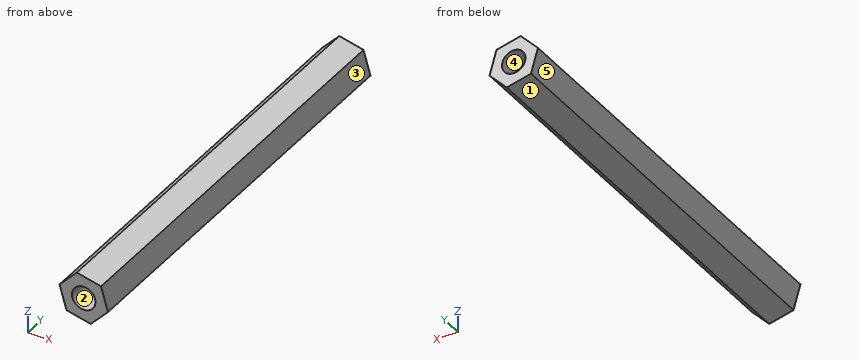
from build123d import *

# Parameters (mm, degrees)
BOSS_EXTRUDE1_DEPTH = 63.5
SKETCH2_R           = 1.7272
CUT_EXTRUDE1_DEPTH  = 9.525
SKETCH3_R           = 1.7272
CUT_EXTRUDE2_DEPTH  = 9.525


with BuildPart() as part:
    # Sketch1 → Boss-Extrude1 (new body)
    with BuildSketch(Plane(origin=(0, 0, 0), x_dir=(1, 0, 0), z_dir=(0, 1, 0))):
        Polygon((-2.767735883, 3.334911674), (-1.744793251, 6.855482892), (-4.282226046, 9.501662807), (-7.842601473, 8.627271504), (-8.865544105, 5.106700285), (-6.32811131, 2.46052037), align=None)
    extrude(amount=BOSS_EXTRUDE1_DEPTH)

    # Sketch2 → Cut-Extrude1 (cut)
    with BuildSketch(Plane(origin=(0, 63.5, 0), x_dir=(1, 0, 0), z_dir=(0, 1, 0))):
        with Locations((-5.305168678, 5.981091589)):
            Circle(SKETCH2_R)
    extrude(amount=-CUT_EXTRUDE1_DEPTH, mode=Mode.SUBTRACT)

    # Sketch3 → Cut-Extrude2 (cut)
    with BuildSketch(Plane.XZ):
        with Locations((-5.305168678, -5.981091589)):
            Circle(SKETCH3_R)
    extrude(amount=-CUT_EXTRUDE2_DEPTH, mode=Mode.SUBTRACT)


solid = part.part
Design review of the part built by this model. Coordinates are the model's own, in mm. Face numbers are marked on the shaded views. A direction names the side the tool comes from. Coordinates: 2 decimals unless noted, no trailing zeros. Order: outer loops, then holes, each group sorted by start corner. A loop starts at its lowest first (then second) coordinate and runs counter-clockwise, first axis right, second up. Notation, with made-up numbers: (2.25, 33) -> (42.25, 33) arc R16 ccw to (42.25, 41) -> close; hole circle Ø4 at (80, -0.5). An arc over 180 degrees is marked (long way). One line per item, written item: value.
1) We need section B-B, the plane x = -5. Give the boundary of the cut face in (y, z) (3 decimals).
Output values:
outline: (0, -9.325) -> (63.5, -9.325) -> (63.5, -7.681) -> (53.975, -7.681) -> (53.975, -4.281) -> (63.5, -4.281) -> (63.5, -2.787) -> (0, -2.787) -> (0, -4.281) -> (9.525, -4.281) -> (9.525, -7.681) -> (0, -7.681) -> close
2) We need section A-A, the plane y = 49.5. Give the boundary of the cut face in (x, z), then the cut area to 3 significant figures.
Output values:
outline: (-8.87, -5.11) -> (-7.84, -8.63) -> (-4.28, -9.5) -> (-1.74, -6.86) -> (-2.77, -3.33) -> (-6.33, -2.46) -> close
area: 34.9 mm2
3) To check wall thickness, follow probe 1 along Y at (x, z) = (-5, -7) (3 decimals); probe 2 along X at (y, z) = (55.5, -7.25); probe 3 along Z at (x, y) = (-6.25, 60.5). State the ranges of each line that lie inside material, in increasing order. Write a range as [from, to].
Output values:
probe 1: y = [9.525, 53.975]
probe 2: x = [-8.24, -6.48], [-4.13, -2.12]
probe 3: z = [-9.02, -7.43], [-4.54, -2.48]
4) Clearance check with flat-ended pins moving along their axes: P1, Ø1, axis at x = -5, z = -6.5, coming from the -Y side (3 decimals); P2, Ø2, axis at x = -5.31, z = -5.98, coming from the +Y side (3 decimals); P3, Ø3, axis at y = 39.5, z = -3.5, coming from the +X side; P4, Ø1.7, axis at x = -4.5, z = -5.5, coming from the +Y side. State where each tip first meets the part, or that it passes through.
Output values:
P1: stops at y = 9.525
P2: stops at y = 53.975
P3: stops at x = -2.28
P4: stops at y = 63.5
5) Draft analysis for pull direction X (two halves, no side actions). For the marked faces 3, 4 and 5, state which applies: +X half, -X half, draft (parallel to the pull), parting line (faces both ways), or undercut.
Output values:
face 3: +X half
face 4: undercut
face 5: -X half
6) Machinability: for the marked faces 1 and 2, which of the approach directions +Z, -Z, +X, -X, +Y, -Y give a long, thin tool a straight path to every point of the face, cutting with its end or side? Answer none if there is none.
Output values:
face 1: -Z, -X, +Y, -Y
face 2: -Y
